The model under review builds one solid part; all positions refer to its coordinate system, in mm. A direction names the side the tool comes from. Round coordinates to 2 decimals unless told otherwise and drop trailing zeros. Order: outer loops, then holes, each group sorted by start corner. A loop starts at its lowest first (then second) coordinate and runs counter-clockwise, first axis right, second up. Notation, with made-up numbers: (34, -34.75) -> (79, -34.75) arc R19 ccw to (79, -11.75) -> close; hole circle Ø5 at (25.25, -16.5). An arc over 180 degrees is marked (long way). Return JSON: item names as keys, results as strings. Group by question number.
from build123d import *

# Parameters (mm, degrees)
BOSS_EXTRUDE1_DEPTH = 3


with BuildPart() as part:
    # Sketch1 → Boss-Extrude1 (new body)
    with BuildSketch(Plane.XY):
        Polygon((0, 0), (0, 7), (3, 7), (3, 14), (0, 14), (0, 21), (3, 21), (3, 28), (0, 28), (0, 35), (3, 35), (3, 42), (0, 42), (0, 50), (-50, 50), (-50, 42), (-53, 42), (-53, 35), (-50, 35), (-50, 28), (-53, 28), (-53, 21), (-50, 21), (-50, 14), (-53, 14), (-53, 7), (-50, 7), (-50, 0), align=None)
        with BuildLine():
            Line((-38.5, 42.5), (-11.5, 42.5))
            ThreePointArc((-11.5, 42.5), (-8.671572875, 41.328427125), (-7.5, 38.5))
            Line((-7.5, 38.5), (-7.5, 38.166666667))
            ThreePointArc((-7.5, 38.166666667), (-8.671572875, 35.338239542), (-11.5, 34.166666667))
            Line((-11.5, 34.166666667), (-38.5, 34.166666667))
            ThreePointArc((-38.5, 34.166666667), (-41.328427125, 35.338239542), (-42.5, 38.166666667))
            Line((-42.5, 38.166666667), (-42.5, 38.5))
            ThreePointArc((-42.5, 38.5), (-41.328427125, 41.328427125), (-38.5, 42.5))
        make_face(mode=Mode.SUBTRACT)
        with BuildLine():
            Line((-38.5, 29.166666667), (-11.5, 29.166666667))
            ThreePointArc((-11.5, 29.166666667), (-8.671572875, 27.995093791), (-7.5, 25.166666667))
            Line((-7.5, 25.166666667), (-7.5, 24.833333333))
            ThreePointArc((-7.5, 24.833333333), (-8.671572875, 22.004906209), (-11.5, 20.833333333))
            Line((-11.5, 20.833333333), (-38.5, 20.833333333))
            ThreePointArc((-38.5, 20.833333333), (-41.328427125, 22.004906209), (-42.5, 24.833333333))
            Line((-42.5, 24.833333333), (-42.5, 25.166666667))
            ThreePointArc((-42.5, 25.166666667), (-41.328427125, 27.995093791), (-38.5, 29.166666667))
        make_face(mode=Mode.SUBTRACT)
        with BuildLine():
            Line((-11.5, 15.833333333), (-38.5, 15.833333333))
            ThreePointArc((-38.5, 15.833333333), (-41.328427125, 14.661760458), (-42.5, 11.833333333))
            Line((-42.5, 11.833333333), (-42.5, 11.5))
            ThreePointArc((-42.5, 11.5), (-41.328427125, 8.671572875), (-38.5, 7.5))
            Line((-38.5, 7.5), (-11.5, 7.5))
            ThreePointArc((-11.5, 7.5), (-8.671572875, 8.671572875), (-7.5, 11.5))
            Line((-7.5, 11.5), (-7.5, 11.833333333))
            ThreePointArc((-7.5, 11.833333333), (-8.671572875, 14.661760458), (-11.5, 15.833333333))
        make_face(mode=Mode.SUBTRACT)
    extrude(amount=BOSS_EXTRUDE1_DEPTH)


solid = part.part
Item 1: Consider section C-C on z = 2.1. Give the number of separate pieces and of enclosed holes in the cut face, plus the area to 3 significant figures.
Item 2: Consider section A-A on x = -35. State the section outline as (y, z) points.
Item 3: Consider section B-B on y = 15. State the section outline as (x, z) points.
Item 4: For faces 4 (the face through (1, 21, 1)), 5 (the face through (-50, 46, 1)), 6 (the face through (-41.359, 8.703, 1.479)), list the 3-axis set-ups (+Z, -Z, +X, -X, +Y, -Y) from which the entire face can be reached by the end or side of a thin tool; tool diameter is ignored.
Item 5: Wall thickness on line 1 along Y through (x, z) = (-33.5, 1.25); line 2 along Y through (x, z) = (1.5, 1.2); line 3 along Y through (x, z) = (-41, 1.1): over which ranges is each line inside the solid? List them lowest first.
Item 6: Consider section D-D on y = 47.5. State the section outline as (x, z) points, plus the area to 3 significant figures.
Item 7: The part is to be moulded in two halves that separate along Y. For faces 1 (the face through (-8.703, 41.359, 1.479)), 2 (the face through (-25, 50, 1)), 3 (the face through (0, 46, 1)), say which applies: +Y half, -Y half, draft (parallel to the pull), parting line (faces both ways), or undercut.
Item 8: Insertion check: pin 1 Ø1.5 at (x, z) = (2, 1) entering from +Y. The pin has a flat end and moves straight along its axis. Give the tip position at first contact, or say it passes through.
Values:
{
 "1": {"separate pieces": "1", "enclosed holes": "3", "area": "1,790 mm^2"},
 "2": {"outline": "(0, 0) -> (7.5, 0) -> (7.5, 3) -> (0, 3) -> close; (15.83, 0) -> (20.83, 0) -> (20.83, 3) -> (15.83, 3) -> close; (29.17, 0) -> (34.17, 0) -> (34.17, 3) -> (29.17, 3) -> close; (42.5, 0) -> (50, 0) -> (50, 3) -> (42.5, 3) -> close"},
 "3": {"outline": "(-50, 0) -> (-40.94, 0) -> (-40.94, 3) -> (-50, 3) -> close; (-9.06, 0) -> (0, 0) -> (0, 3) -> (-9.06, 3) -> close"},
 "4": {"face 4": "+Z, -Z, +X", "face 5": "+Z, -Z, -X, +Y", "face 6": "+Z, -Z"},
 "5": {"line 1": "0 to 7.5, 15.83 to 20.83, 29.17 to 34.17, 42.5 to 50", "line 2": "7 to 14, 21 to 28, 35 to 42", "line 3": "0 to 8.38, 14.96 to 21.71, 28.29 to 35.04, 41.62 to 50"},
 "6": {"outline": "(-50, 0) -> (0, 0) -> (0, 3) -> (-50, 3) -> close", "area": "150 mm^2"},
 "7": {"face 1": "undercut", "face 2": "+Y half", "face 3": "draft"},
 "8": {"pin 1": "y = 42"}
}
